Read the model definition and answer for the solid it produces. Units are mm, in the model's axes. A direction names the side the tool comes from. Coordinates: 2 decimals unless noted, no trailing zeros. Loops run counter-clockwise (first coordinate to the right, second up) from the corner with the lowest first, then second, coordinate; pieces in that order, holes last. Notation, with made-up numbers: M 69,55.25 L 126,55.25 A12 ccw 126,74.25 Z; hole C 59.5,-18.5 d5. An arc over 180 degrees is marked long. Put each result on its own line as item: value.
from build123d import *

# Parameters (mm, degrees)
SKETCH_W        = 52
SKETCH_H        = 21
SKETCH_R        = 3
PAD_DEPTH       = 3
SKETCH001_W     = 29
SKETCH001_H     = 14
SKETCH001_R     = 1.5
PAD001_DEPTH    = 11
POCKET_DEPTH    = 100
PAD002_DEPTH    = 29
SKETCH004_W     = 3.506214
SKETCH004_H     = 4.561438
SKETCH004_W_2   = 13.343595
SKETCH004_H_2   = 5.385539
SKETCH004_W_3   = 3.315279
SKETCH004_H_3   = 4.172676
POCKET001_DEPTH = 7


with BuildPart() as part:
    # Sketch → Pad (new body)
    with BuildSketch(Plane.XY):
        with Locations((26, 10.5)):
            Rectangle(SKETCH_W, SKETCH_H)
        with Locations((5.25, 10.5)):
            Circle(SKETCH_R, mode=Mode.SUBTRACT)
        with Locations((46.75, 10.498532)):
            Circle(SKETCH_R, mode=Mode.SUBTRACT)
    extrude(amount=PAD_DEPTH)

    # Sketch001 → Pad001 (new body)
    with BuildSketch(Plane.XY.offset(3)):
        with Locations((25.906526, 10)):
            Rectangle(SKETCH001_W, SKETCH001_H)
        with Locations((16.906526, 7)):
            Circle(SKETCH001_R, mode=Mode.SUBTRACT)
        with Locations((34.906526, 7)):
            Circle(SKETCH001_R, mode=Mode.SUBTRACT)
    extrude(amount=PAD001_DEPTH)

    # Sketch002 → Pocket (cut)
    with BuildSketch(Plane.YZ.offset(40.406526)):
        with BuildLine():
            ThreePointArc((17, 3.044285), (15.003799, 9.482974), (10, 14))
            Line((10, 14), (17, 14))
            Line((17, 14), (17, 3.044285))
        make_face()
    extrude(amount=-POCKET_DEPTH, mode=Mode.SUBTRACT)

    # Sketch003 → Pad002 (new body)
    with BuildSketch(Plane.YZ.offset(40.406526)):
        with BuildLine():
            Line((8.354331, 14.091598), (8.354331, 13.391598))
            ThreePointArc((8.354331, 13.391598), (12.257184, 14.090805), (15.354331, 16.566454))
            Line((14.840477, 17.041801), (15.354331, 16.566454))
            ThreePointArc((8.354331, 14.091598), (11.93941, 14.814785), (14.840477, 17.041801))
        make_face()
    extrude(amount=-PAD002_DEPTH)

    # Sketch004 → Pocket001 (cut)
    with BuildSketch(Plane.XZ.offset(-8.354331)):
        with Locations((38.987986, 15.672686)):
            Rectangle(SKETCH004_W, SKETCH004_H)
        with Locations((25.624218, 16.18705)):
            Rectangle(SKETCH004_W_2, SKETCH004_H_2)
        with Locations((12.72779, 15.529459)):
            Rectangle(SKETCH004_W_3, SKETCH004_H_3)
    extrude(amount=-POCKET001_DEPTH, mode=Mode.SUBTRACT)


solid = part.part
1) Determine the mould class of faces 1 (the flat face through (26, 0, 1)), 2 (the flat face through (40.407, 8, 9)), 3 (the flat face through (32.296, 11.84, 14.6)) for opening direction X: released by +X, released by -X, zero draft, split by the parting line, or undercut.
Answer list:
face 1: zero draft
face 2: released by +X
face 3: undercut
2) Find section D-D, the plane y = 12.5. Write down the section's boundary in (x, z).
Answer list:
outline: M 0,0 L 3.01,0 L 3.01,3 L 0,3 Z; M 7.49,0 L 44.52,0 L 44.52,3 L 40.41,3 L 40.41,12.35 L 11.41,12.35 L 11.41,3 L 7.49,3 Z; M 14.39,14.21 L 18.95,14.21 L 18.95,15.1 L 14.39,15.1 Z; M 32.3,14.21 L 37.23,14.21 L 37.23,15.1 L 32.3,15.1 Z; M 48.98,0 L 52,0 L 52,3 L 48.98,3 Z
3) Given pin 1 Ø1.5 at (x, y) = (7.5, 7.5) entering from +Z; pin 2 Ø1.6 at (x, y) = (29.5, 4.5) entering from +Z; pin 3 Ø3.5 at (x, y) = (16, 7.5) entering from +Z, each flat-ended and moving along its own axis, determine where each tip first touches the part or whether it passes through.
Answer list:
pin 1: stops at z = 3
pin 2: stops at z = 14
pin 3: stops at z = 14.12
4) Find section C-C, the plane x = 30.5. Write down the section's boundary in (y, z), plus the area to 3 significant figures.
Answer list:
outline: M 0,0 L 21,0 L 21,3 L 17,3 L 17,3.04 A12.73 ccw 10.91,13.49 L 8.35,13.49 L 8.35,14 L 3,14 L 3,3 L 0,3 Z
area: 193 mm^2
5) Find section A-A, the plane x = 46.75. Write down the section's boundary in (y, z).
Answer list:
outline: M 0,0 L 7.5,0 L 7.5,3 L 0,3 Z; M 13.5,0 L 21,0 L 21,3 L 13.5,3 Z
6) Which of the six approach directions +Z, -Z, +X, -X, +Y, -Y give full straight-line access (tool end or side, diameter ignored) to faces 4 (the flat face through (18.952, 11.84, 14.6)), 5 (the flat face through (13, 10, 13.443)), 6 (the flat face through (11.407, 8, 9))?
Answer list:
face 4: +Z, +Y
face 5: +Z, -X, +Y
face 6: +Z, -X, +Y, -Y
7) Find section B-B, the plane y = 4. Write down the section's boundary in (x, z), plus the area to 3 significant figures.
Answer list:
outline: M 0,0 L 52,0 L 52,3 L 40.41,3 L 40.41,14 L 11.41,14 L 11.41,3 L 0,3 Z
area: 475 mm^2
8) Straight lines are drawn through the part: line 1 (X direction, y = 7, z = 7); line 2 (Y direction, x = 46.75, z = 1.3); line 3 (X direction, y = 12.5, z = 0.5). For each, find the intervals that lie inside material, in ascending order. Write a range as [from, to].
Answer list:
line 1: x = [11.41, 15.41], [18.41, 33.41], [36.41, 40.41]
line 2: y = [0, 7.5], [13.5, 21]
line 3: x = [0, 3.01], [7.49, 44.52], [48.98, 52]
